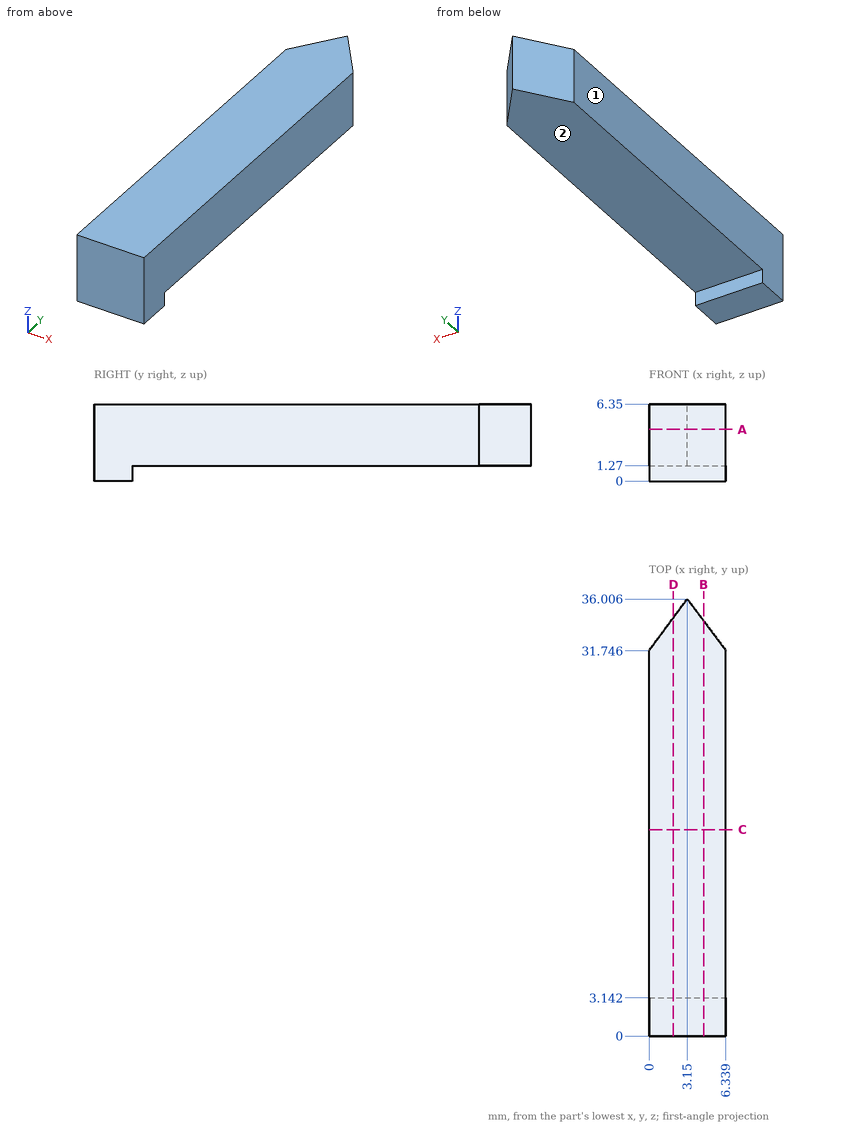
Here's the drawing with two shaded views (mm, measured from the low corner). I have some questions. A direction names the side the tool comes from. Round coordinates to 2 decimals unless told otherwise and drop trailing zeros. Loops run counter-clockwise (first coordinate to the right, second up) from the corner with the lowest first, then second, coordinate; pieces in that order, holes last. Notation, with made-up numbers: (37.5, -37.5) - (80.5, -37.5) arc R20 cw to (80.5, -24.5) - close; hole circle Ø11 at (28, -30). An arc over 180 degrees is marked (long way). Write item = value, one per line.
1) Imagine slicing it at C-C (y = 17). Please give me the cut outline in (x, z).
Computed:
outline = (0, 1.27) - (6.34, 1.27) - (6.34, 6.35) - (0, 6.35) - close
2) Imagine slicing it at D-D (x = 2). Please give me the cut outline in (y, z), and give its area (3 significant figures).
Computed:
outline = (0, 0) - (3.14, 0) - (3.14, 1.27) - (34.45, 1.27) - (34.45, 6.35) - (0, 6.35) - close
area = 179 mm2
3) On a 3-axis mill with a long thin cutter (end or side, diameter ignored), from which of +Z, -Z, +X, -X, +Y, -Y can I reach the whole of each face in a straight line? I mean the marked faces 1 and 2. Say none if no direction works.
Computed:
face_1 = +Z, -Z, -X, +Y, -Y
face_2 = -Z, +X, -X, +Y
4) I'm going to push a flat-ended pin straight in: P1, Ø3, axis at x = 2, y = 22.5, coming from the -Z side. Where does the tip first touch, or does it pass through?
Computed:
P1 = 1.27
5) I need wall thicknesses on line 1 along Z through (x, y) = (1.75, 26.5); line 2 along Y through (x, z) = (0.5, 0.75); line 3 along Y through (x, z) = (5, 5) (1 decimal). Which ranges of each line are inside material? Lowest first, please. Write a range as from..to.
Computed:
line_1 = 1.27..6.35
line_2 = 0..3.14
line_3 = 0..33.5
6) Imagine slicing it at A-A (z = 4.25). Please give me the cut outline in (x, y), and give its area (3 significant figures).
Computed:
outline = (0, 0) - (6.34, 0) - (6.34, 31.75) - (3.15, 36.01) - (0, 31.75) - close
area = 215 mm2
7) Imagine slicing it at B-B (x = 4.5). Please give me the cut outline in (y, z), and give its area (3 significant figures).
Computed:
outline = (0, 0) - (3.14, 0) - (3.14, 1.27) - (34.2, 1.27) - (34.2, 6.35) - (0, 6.35) - close
area = 178 mm2
